from build123d import *

# Parameters (mm, degrees)
BOSS_EXTRUDE1_DEPTH = 300
SKETCH2_W           = 10
SKETCH2_H           = 10
BOSS_EXTRUDE2_DEPTH = 2
SKETCH4_R           = 15
SKETCH4_R_2         = 14
SKETCH4_R_3         = 10
BOSS_EXTRUDE3_DEPTH = 2
SKETCH4_3_R         = 10
CUT_EXTRUDE1_DEPTH  = 2


with BuildPart() as part:
    # Sketch1 → Boss-Extrude1 (new body)
    with BuildSketch(Plane(origin=(0, 0, 0), x_dir=(0, 0, -1), z_dir=(1, 0, 0))):
        with BuildLine():
            Line((10, 13), (10, -13))
            ThreePointArc((10, -13), (9.414213562, -14.414213562), (8, -15))
            Line((8, -15), (0, -15))
            Line((0, -15), (0, -14))
            Line((0, -14), (7, -14))
            ThreePointArc((7, -14), (8.414213562, -13.414213562), (9, -12))
            Line((9, -12), (9, 12))
            ThreePointArc((9, 12), (8.414213562, 13.414213562), (7, 14))
            Line((7, 14), (0, 14))
            Line((0, 14), (0, 15))
            Line((0, 15), (8, 15))
            ThreePointArc((8, 15), (9.414213562, 14.414213562), (10, 13))
        make_face()
    extrude(amount=BOSS_EXTRUDE1_DEPTH)

    # Sketch2 → Boss-Extrude2 (add)
    with BuildSketch(Plane.XY):
        with Locations((75, 20)):
            Rectangle(SKETCH2_W, SKETCH2_H)
        with Locations((75, -20)):
            Rectangle(SKETCH2_W, SKETCH2_H)
        with Locations((225, 20)):
            Rectangle(SKETCH2_W, SKETCH2_H)
        with Locations((225, -20)):
            Rectangle(SKETCH2_W, SKETCH2_H)
    extrude(amount=-BOSS_EXTRUDE2_DEPTH)

    # Sketch4 → Boss-Extrude3 (add)
    # profile 1 of 2: a face of its own
    with BuildSketch(Plane(origin=(0, 0, -10), x_dir=(-1, 0, 0), z_dir=(0, 0, -1))):
        Circle(SKETCH4_R)
        Circle(SKETCH4_R_2, mode=Mode.SUBTRACT)
    # profile 2 of 2: a face of its own
    with BuildSketch(Plane(origin=(0, 0, -10), x_dir=(-1, 0, 0), z_dir=(0, 0, -1))):
        Circle(SKETCH4_R_2)
        with Locations(Location((0, 0, 0), (0, 0, 90))):
            Circle(SKETCH4_R_3, mode=Mode.SUBTRACT)
    extrude(amount=-BOSS_EXTRUDE3_DEPTH)

    # Sketch4_3 → Cut-Extrude1 (cut)
    with BuildSketch(Plane(origin=(0, 0, -10), x_dir=(-1, 0, 0), z_dir=(0, 0, -1))):
        with Locations(Location((0, 0, 0), (0, 0, 90))):
            Circle(SKETCH4_3_R)
    extrude(amount=-CUT_EXTRUDE1_DEPTH, mode=Mode.SUBTRACT)


solid = part.part
For this review, take the finished solid that the model builds, in its own axes (mm). A direction names the side the tool comes from. Coordinates: 2 decimals unless noted, no trailing zeros. Loops run counter-clockwise (first coordinate to the right, second up) from the corner with the lowest first, then second, coordinate; pieces in that order, holes last. Notation, with made-up numbers: (46, -8) - (75, -8) arc R17 ccw to (75, 3) - close; hole circle Ø6 at (64.5, 84). An arc over 180 degrees is marked (long way). Use a Markdown table: item, result. Add a question column.
Item 1: Tool access review of faces 1 (the face through (225, -20, -2)), 2 (the face through (145, 0, -10)), 3 (the face through (152, 0, -9)), 4 (the face through (148, 14, -4)), 5 (the face through (75, 20, -2)): name each direction out of +Z, -Z, +X, -X, +Y, -Y from which nothing blocks a thin tool from reaching the whole face with its end or side.
Item 2: We need section C-C (x = 239). Give the boundary of the cut face in (y, z), and give its area (3 significant figures).
Item 3: We need section B-B (z = -3.75). Give the boundary of the cut face in (x, y), and give its area (3 significant figures).
Item 4: We need section A-A (y = 0). Give the boundary of the cut face in (x, z).
Item 5: Insertion check: pin 1 Ø3 at (x, z) = (148, -6.5) entering from -Y; pin 2 Ø2 at (y, z) = (21, -0.5) entering from -X; pin 3 Ø4 at (y, z) = (12.5, -9) entering from -X. Each pin has a flat end and moves straight along its axis. Give the tip position at first contact, or say it passes through.
Item 6: For line 1 (Y direction, x = 129.5, z = -6.25); line 2 (X direction, y = 20, z = -1); line 3 (Y direction, x = 0, z = -9), list the stretches that pass through material, from the lowest coordinate up.
Item 7: Mouldability with a two-part tool opening along X and no side actions: class faces 6 (the face through (300, 1.2, -9.5)), 7 (the face through (148, 15, -4)), 8 (the face through (149.3, -14.6, 0)) as pulls with the +X half, pulls with the -X half, needs draft (parallel to the pull), parting line crosses it, or undercut.
Results list:
| question | item | result |
|---|---|---|
| 1 | face 1 | -Z, +X, -X, -Y |
| 1 | face 2 | -Z, +X, -X, +Y, -Y |
| 1 | face 3 | +Z, +X |
| 1 | face 4 | +Z, +X, -X |
| 1 | face 5 | -Z, +X, -X, +Y |
| 2 | outline | (-15, -8) arc R2 ccw to (-13, -10) - (13, -10) arc R2 ccw to (15, -8) - (15, 0) - (14, 0) - (14, -7) arc R2 cw to (12, -9) - (-12, -9) arc R2 cw to (-14, -7) - (-14, 0) - (-15, 0) - close |
| 2 | area | 48.0 mm^2 |
| 3 | outline | (0, -15) - (300, -15) - (300, -14) - (0, -14) - close; (0, 14) - (300, 14) - (300, 15) - (0, 15) - close |
| 3 | area | 600 mm^2 |
| 4 | outline | (-15, -10) - (-10, -10) - (-10, -8) - (-15, -8) - close; (10, -10) - (300, -10) - (300, -9) - (15, -9) - (15, -8) - (10, -8) - close |
| 5 | pin 1 | stops at y = -15 |
| 5 | pin 2 | stops at x = 70 |
| 5 | pin 3 | stops at x = -10.71 |
| 6 | line 1 | y = -15 to -14, 14 to 15 |
| 6 | line 2 | x = 70 to 80, 220 to 230 |
| 6 | line 3 | y = -15 to -10, 10 to 15 |
| 7 | face 6 | pulls with the +X half |
| 7 | face 7 | undercut |
| 7 | face 8 | needs draft |
